from build123d import *

# Parameters (mm, degrees)
SKETCH1_W                   = 110
SKETCH1_H                   = 34
BOSS_EXTRUDE1_DEPTH         = 6.35
M5_CLEARANCE_HOLE1_D        = 5.8
TAP_DRILL_FOR_M5X0_8_TAP1_D = 4.2
CUT_EXTRUDE1_DEPTH          = 77.299230009
CUT_EXTRUDE2_DEPTH          = 1.87


with BuildPart() as part:
    # Sketch1 → Boss-Extrude1 (new body)
    with BuildSketch(Plane.XZ):
        with Locations((13.5, 16)):
            Rectangle(SKETCH1_W, SKETCH1_H)
    extrude(amount=-BOSS_EXTRUDE1_DEPTH)

    # M5 Clearance Hole1 (through all)
    with Locations(Plane(origin=(0, 6.35, 0), x_dir=(1, 0, 0), z_dir=(0, 1, 0))):
        with Locations((-35.5, -5.5), (-7.5, -5.5), (7.5, -5.5), (35.5, -5.5), (-35.5, -26.5), (-7.5, -26.5), (7.5, -26.5), (35.5, -26.5)):
            Hole(M5_CLEARANCE_HOLE1_D / 2)

    # Tap Drill for M5x0.8 Tap1 (through all)
    with Locations(Plane(origin=(0, 6.35, 0), x_dir=(1, 0, 0), z_dir=(0, 1, 0))):
        with Locations((-18.5, -16), (18.5, -16)):
            Hole(TAP_DRILL_FOR_M5X0_8_TAP1_D / 2)

    # Sketch9 → Cut-Extrude1 (cut, through all)
    with BuildSketch(Plane(origin=(0, 6.35, 0), x_dir=(1, 0, 0), z_dir=(0, 1, 0))):
        with BuildLine():
            Line((68.5, -10.1), (58.5, -10.1))
            ThreePointArc((58.5, -10.1), (53.949193338, -16), (58.5, -21.9))
            Line((58.5, -21.9), (68.5, -21.9))
            Line((68.5, -21.9), (68.5, -10.1))
        make_face()
    extrude(amount=-CUT_EXTRUDE1_DEPTH, mode=Mode.SUBTRACT)

    # Sketch10 → Cut-Extrude2 (cut)
    with BuildSketch(Plane(origin=(0, 0, 0), x_dir=(1, 0, 0), z_dir=(0, 1, 0))):
        with BuildLine():
            Line((68.5, -24.25), (60.049193338, -24.25))
            ThreePointArc((60.049193338, -24.25), (51.799193338, -16), (60.049193338, -7.75))
            Line((60.049193338, -7.75), (68.5, -7.75))
            Line((68.5, -7.75), (68.5, -24.25))
        make_face()
    extrude(amount=CUT_EXTRUDE2_DEPTH, mode=Mode.SUBTRACT)


solid = part.part
The model under review builds one solid part; all positions refer to its coordinate system, in mm. A direction names the side the tool comes from. Give positions to 0.01 mm unless a question says otherwise; leave off trailing zeros. Order: outer loops, then holes, each group sorted by start corner. A loop starts at its lowest first (then second) coordinate and runs counter-clockwise, first axis right, second up. Notation, with made-up numbers: M 18,29.25 L 40,29.25 A25 cw 40,65.25 Z; hole C -15,-20.75 d2. An arc over 180 degrees is marked long. One line per question, with ' | ' between items. Start each with the question number.
1) For faces 1 (the face through (64, 4, 10.1)), 2 (the face through (51.8, 0.9, 16.2)), 3 (the face through (68.5, 3, 4)), list the 3-axis set-ups (+Z, -Z, +X, -X, +Y, -Y) from which the entire face can be reached by the end or side of a thin tool; tool diameter is ignored.
2) Wall thickness on L1, parallel to X at y = 4.5, z = 26.5; L2, parallel to Z at x = 7.5, y = 3.5; L3, parallel to Z at x = 64, y = 3.75: over which ranges is each line inside the solid? List them lowest first. Write a range as from..to.
3) Consider section A-A, the plane z = 16. Give the boundary of the cut face in (x, y).
4) Consider section B-B, the plane x = 35.5. Give the boundary of the cut face in (y, z).
5) Mouldability with a two-part tool opening along Z and no side actions: class faces 4 (the face through (13, 3, -1)), 5 (the face through (9.801, 3.131, 28.265)), 6 (the face through (-41.5, 3, 16)) as pulls with the +Z half, pulls with the -Z half, needs draft (parallel to the pull), parting line crosses it, or undercut.
6) Consider section D-D, the plane y = 5. State how many separate pieces and enclosed holes the cut face has, then the cut area to 3 significant figures.
7) Consider section C-C, the plane x = -18.5. Give the boundary of the cut face in (y, z), then the cut area to 3 significant figures.
Found:
1) face 1: +X, +Y, -Y | face 2: +X, -Y | face 3: +Z, -Z, +X, +Y, -Y
2) L1: x = -41.5..-38.4, -32.6..-10.4, -4.6..4.6, 10.4..32.6, 38.4..68.5 | L2: z = -1..2.6, 8.4..23.6, 29.4..33 | L3: z = -1..10.1, 21.9..33
3) outline: M -41.5,0 L -20.6,0 L -20.6,6.35 L -41.5,6.35 Z; M -16.4,0 L 16.4,0 L 16.4,6.35 L -16.4,6.35 Z; M 20.6,0 L 51.8,0 L 51.8,1.87 L 53.95,1.87 L 53.95,6.35 L 20.6,6.35 Z
4) outline: M 0,-1 L 6.35,-1 L 6.35,2.6 L 0,2.6 Z; M 0,8.4 L 6.35,8.4 L 6.35,23.6 L 0,23.6 Z; M 0,29.4 L 6.35,29.4 L 6.35,33 L 0,33 Z
5) face 4: pulls with the -Z half | face 5: undercut | face 6: needs draft
6) separate pieces: 1 | enclosed holes: 10 | area: 3,340 mm²
7) outline: M 0,-1 L 6.35,-1 L 6.35,13.9 L 0,13.9 Z; M 0,18.1 L 6.35,18.1 L 6.35,33 L 0,33 Z | area: 189 mm²
